from build123d import *

# Parameters (mm, degrees)
F1_DEPTH    = 27.94
F3_DEPTH    = 50.8
F4_T1_DEPTH = 44.9110888614
F5_R        = 2.54
F6_W        = 15.24
F6_H        = 2.032
F7_DEPTH    = 25.4
F9_DEPTH    = 5.08
F10_DEPTH   = 5.08


# Not quite as in the source:
# - a fillet or chamfer that OpenCascade refuses, or shapes differently, is made with other operations: its cross-section is extruded or revolved along the edge and cut away or added


with BuildPart() as f1:
    # F0 (on Front) → F1 (new body)
    with BuildSketch(Plane.XZ):
        with BuildLine():
            ThreePointArc((-4.445, -11.8967211869), (-12.3269517561, -3.0555294801), (-9.4867838955, 8.4433957221))
            Line((-9.4867838955, 8.4433957221), (-11.3841406746, 10.1320748666))
            ThreePointArc((-11.3841406746, 10.1320748666), (-15.1860134607, -1.281637691), (-9.525, -11.8967211869))
            Line((-9.525, -11.8967211869), (-4.445, -11.8967211869))
        make_face()
        with BuildLine():
            Line((9.525, -11.8967211869), (4.445, -11.8967211869))
            ThreePointArc((4.445, -11.8967211869), (0, -12.7), (-4.445, -11.8967211869))
            Line((-4.445, -11.8967211869), (-9.525, -11.8967211869))
            ThreePointArc((-9.525, -11.8967211869), (0, -15.24), (9.525, -11.8967211869))
        make_face()
        with BuildLine():
            Line((9.525, -25.4), (9.525, -11.8967211869))
            ThreePointArc((9.525, -11.8967211869), (0, -15.24), (-9.525, -11.8967211869))
            Line((-9.525, -11.8967211869), (-9.525, -25.4))
            Line((-9.525, -25.4), (9.525, -25.4))
        make_face()
        with BuildLine():
            ThreePointArc((8.4433957221, 9.4867838955), (11.5870860373, 5.1989842435), (12.7, 0))
            ThreePointArc((12.7, 0), (10.4341147205, -7.2401139494), (4.445, -11.8967211869))
            Line((4.445, -11.8967211869), (9.525, -11.8967211869))
            ThreePointArc((9.525, -11.8967211869), (13.7371503595, -6.5991135768), (15.24, 0))
            ThreePointArc((15.24, 0), (13.9045032448, 6.2387810922), (10.1320748666, 11.3841406746))
            Line((10.1320748666, 11.3841406746), (8.4433957221, 9.4867838955))
        make_face()
    extrude(amount=F1_DEPTH)

    # F2 (on face) → F3 (join)
    with BuildSketch(Plane(origin=(0, 0, -25.4), x_dir=(1, 0, 0), z_dir=(0, 0, -1))):
        with BuildLine():
            Line((-9.525, 0), (-4.2597094971, 0))
            ThreePointArc((-4.2597094971, 0), (-7.0430625309, 1.175419304), (-9.525, 2.8983966834))
            Line((-9.525, 2.8983966834), (-9.525, 0))
        make_face()
        with BuildLine():
            Line((9.525, 2.8983966834), (9.525, 25.0416033166))
            ThreePointArc((9.525, 25.0416033166), (7.0430625309, 26.764580696), (4.2597094971, 27.94))
            Line((4.2597094971, 27.94), (-4.2597094971, 27.94))
            ThreePointArc((-4.2597094971, 27.94), (-7.0430625309, 26.764580696), (-9.525, 25.0416033166))
            Line((-9.525, 25.0416033166), (-9.525, 2.8983966834))
            ThreePointArc((-9.525, 2.8983966834), (-7.0430625309, 1.175419304), (-4.2597094971, 0))
            Line((-4.2597094971, 0), (4.2597094971, 0))
            ThreePointArc((4.2597094971, 0), (7.0430625309, 1.175419304), (9.525, 2.8983966834))
        make_face()
        with BuildLine():
            Line((9.525, 0), (9.525, 2.8983966834))
            ThreePointArc((9.525, 2.8983966834), (7.0430625309, 1.175419304), (4.2597094971, 0))
            Line((4.2597094971, 0), (9.525, 0))
        make_face()
        with BuildLine():
            ThreePointArc((-9.525, 25.0416033166), (-7.0430625309, 26.764580696), (-4.2597094971, 27.94))
            Line((-4.2597094971, 27.94), (-9.525, 27.94))
            Line((-9.525, 27.94), (-9.525, 25.0416033166))
        make_face()
        with BuildLine():
            ThreePointArc((4.2597094971, 27.94), (7.0430625309, 26.764580696), (9.525, 25.0416033166))
            Line((9.525, 25.0416033166), (9.525, 27.94))
            Line((9.525, 27.94), (4.2597094971, 27.94))
        make_face()
    extrude(amount=F3_DEPTH)

    # F4: fillet of radius 5.08 on 2 edges, made by hand

    # F4_s2 → F4_t1 (cut)
    with BuildSketch(Plane.XZ.offset(-8.4855444307)):
        with BuildLine():
            ThreePointArc((-11.3841406746, 10.1320748666), (-10.8580531921, 7.8805841193), (-11.3843237056, 5.6291361473))
            ThreePointArc((-11.3843237056, 5.6291361473), (-10.5299951264, 7.0999438475), (-9.4867838955, 8.4433957221))
            Line((-9.4867838955, 8.4433957221), (-11.3841406746, 10.1320748666))
        make_face()
        with BuildLine():
            ThreePointArc((10.1320748666, 11.3841406746), (9.8706902669, 9.0868255644), (10.6545556025, 6.9116166642))
            ThreePointArc((10.6545556025, 6.9116166642), (9.6353934931, 8.2734026998), (8.4433957221, 9.4867838955))
            Line((8.4433957221, 9.4867838955), (10.1320748666, 11.3841406746))
        make_face()
    extrude(amount=F4_T1_DEPTH, mode=Mode.SUBTRACT)

    # F5
    f5_edges = [f1.edges().sort_by_distance(p)[0] for p in [
        (-9.525, -27.94, -44.048361),
        (9.525, -27.94, -44.048361),
    ]]
    fillet(f5_edges, radius=F5_R)

    # F6 (on face) → F7 (cut)
    with BuildSketch(Plane.YZ.offset(9.525)):
        with Locations((-13.1727202785, -17.1660094585)):
            Rectangle(F6_W, F6_H)
    extrude(amount=-F7_DEPTH, mode=Mode.SUBTRACT)

    # F8 (on face) → F9 (join)
    with BuildSketch(Plane(origin=(0, 0, -76.2), x_dir=(1, 0, 0), z_dir=(0, 0, -1))):
        with BuildLine():
            ThreePointArc((9.525, 3.3432788131), (13.7371503595, 8.6408864232), (15.24, 15.24))
            ThreePointArc((15.24, 15.24), (-6.5991135768, 28.9771503595), (-9.525, 3.3432788131))
            Line((-9.525, 3.3432788131), (-9.525, 25.4))
            ThreePointArc((-9.525, 25.4), (-8.7810512242, 27.1960512242), (-6.985, 27.94))
            Line((-6.985, 27.94), (6.985, 27.94))
            ThreePointArc((6.985, 27.94), (8.7810512242, 27.1960512242), (9.525, 25.4))
            Line((9.525, 25.4), (9.525, 3.3432788131))
        make_face()
        with BuildLine():
            Line((-9.525, 25.4), (-9.525, 3.3432788131))
            ThreePointArc((-9.525, 3.3432788131), (-5.0473542134, 0.8600898666), (0, 0))
            ThreePointArc((0, 0), (5.0473542134, 0.8600898666), (9.525, 3.3432788131))
            Line((9.525, 3.3432788131), (9.525, 25.4))
            ThreePointArc((9.525, 25.4), (8.7810512242, 27.1960512242), (6.985, 27.94))
            Line((6.985, 27.94), (-6.985, 27.94))
            ThreePointArc((-6.985, 27.94), (-8.7810512242, 27.1960512242), (-9.525, 25.4))
        make_face()
    extrude(amount=F9_DEPTH)

    # F10 (add): faces of the model
    f10_faces = [f1.faces().sort_by_distance(p)[0] for p in [
        (-7.1991537336, -0.9808264472, -76.2),
        (7.1991537336, -0.9808264472, -76.2),
    ]]
    extrude(f10_faces, amount=F10_DEPTH)


solid = f1.part
Geometry: final body of the model. Coordinates: model frame, mm. A direction names the side the tool comes from. Give positions to 0.01 mm unless a question says otherwise; leave off trailing zeros. Order: outer loops, then holes, each group sorted by start corner. A loop starts at its lowest first (then second) coordinate and runs counter-clockwise, first axis right, second up. Notation, with made-up numbers: (72, 14) -> (81, 14) arc R20 ccw to (81, 39) -> close; hole circle Ø8 at (-20.5, 82). An arc over 180 degrees is marked (long way). Write each question's results on one line, items separated by ' | '.
1) First-contact query: pin 1 Ø10 at (y, z) = (-14.5, -23) entering from -X (3 decimals); pin 2 Ø8 at (y, z) = (-10.5, -40) entering from +X (3 decimals); pin 3 Ø12 at (x, y) = (-4, -10) entering from +Z. Flat tips, straight axial feed; report the tip coordinate or a pass-through.
Geometry says:
pin 1: stops at x = -9.525 | pin 2: stops at x = 9.525 | pin 3: stops at z = -7.83
2) Draft query along Y for faces 5 (the face through (0, -15, -81.28)), 6 (the face through (0, -5.553, -17)), 7 (the face through (0, 0, -45)). Return one class per face: released by +Y, released by -Y, zero draft, split by the parting line, or undercut.
Geometry says:
face 5: zero draft | face 6: undercut | face 7: released by +Y
3) Cut plane B-B (z = -8). Output: boundary loops of the cut face in (x, y), and give its area (3 significant figures).
Geometry says:
outline: (-12.97, -27.94) -> (-9.86, -27.94) -> (-9.86, 0) -> (-12.97, 0) -> close; (9.86, -27.94) -> (12.97, -27.94) -> (12.97, 0) -> (9.86, 0) -> close | area: 174 mm²
4) Line query: line 1 along Z through (x, y) = (10.5, -23.5); line 2 along Y through (x, z) = (3.5, -35); line 3 along Z through (x, y) = (-2, -17). Output: solid intervals per line, ascending.
Geometry says:
line 1: z = -81.28 to -76.2, -11.05 to -7.14, 7.17 to 11.05 | line 2: y = -27.94 to 0 | line 3: z = -81.28 to -18.18, -16.15 to -12.54
5) Cut plane D-D (y = -24.5). Output: boundary loops of the cut face in (x, z) (3 decimals).
Geometry says:
outline: (-12.104, -81.28) -> (12.104, -81.28) -> (12.104, -76.2) -> (9.525, -76.2) -> (9.525, -11.897) arc R15.24 ccw to (10.132, 11.384) arc R5.08 ccw to (10.655, 6.912) arc R12.7 cw (long way) to (-11.384, 5.629) arc R5.08 ccw to (-11.384, 10.132) arc R15.24 ccw to (-9.525, -11.897) -> (-9.525, -76.2) -> (-12.104, -76.2) -> close
6) Cut plane C-C (z = -36). Output: boundary loops of the cut face in (x, y) (3 decimals).
Geometry says:
outline: (-9.525, -25.4) arc R2.54 ccw to (-6.985, -27.94) -> (6.985, -27.94) arc R2.54 ccw to (9.525, -25.4) -> (9.525, 0) -> (-9.525, 0) -> close
7) Set-up query: faces 1 (the face through (9.867, -13.774, 9.119)), 2 (the face through (8.801, -27.176, -44.498)), 3 (the face through (0, -13, -16.15)), 4 (the face through (-3, -27.94, -42)). Return all of +Z, -Z, +X, -X, +Y, -Y with unobstructed straight access to the full face (end or side cutting, diameter ignored); none if empty.
Geometry says:
face 1: +Y, -Y | face 2: +X, -Y | face 3: +X, -X | face 4: +Z, +X, -X, -Y
8) Cut plane A-A (x = 0). Output: boundary loops of the cut face in (y, z).
Geometry says:
outline: (-30.48, -81.28) -> (0, -81.28) -> (0, -12.7) -> (-27.94, -12.7) -> (-27.94, -76.2) -> (-30.48, -76.2) -> close; hole (-20.79, -18.18) -> (-5.55, -18.18) -> (-5.55, -16.15) -> (-20.79, -16.15) -> close
